```python
from build123d import *

# Parameters (mm, degrees)
SKETCH1_W                      = 260
SKETCH1_H                      = 132
BOSS_EXTRUDE1_DEPTH            = 150
SHELL1_T                       = -12
SKETCH2_W                      = 270
SKETCH2_H                      = 160
SKETCH2_W_2                    = 260
SKETCH2_H_2                    = 132
BOSS_EXTRUDE2_DEPTH            = 10
SKETCH3_R                      = 3.5
CUT_EXTRUDE1_DEPTH             = 10
CUT_EXTRUDE2_REACH             = 251.08
SKETCH4_R                      = 21
CHAMFER1_SIZE                  = 1
FILLET1_R                      = 2
M5_CLEARANCE_HOLE1_D           = 5.3
M5_CLEARANCE_HOLE1_CSINK_D     = 5.35
M5_CLEARANCE_HOLE1_CSINK_ANGLE = 90


with BuildPart() as part:
    # Sketch1 → Boss-Extrude1 (new body)
    with BuildSketch(Plane(origin=(0, 0, 0), x_dir=(1, 0, 0), z_dir=(0, 1, 0))):
        Rectangle(SKETCH1_W, SKETCH1_H)
    extrude(amount=BOSS_EXTRUDE1_DEPTH)

    # Shell1
    shell1_openings = [part.faces().sort_by_distance(p)[0] for p in [
        (0, 150, 0),
    ]]
    offset(amount=SHELL1_T, openings=shell1_openings, kind=Kind.INTERSECTION)

    # Sketch2 → Boss-Extrude2 (add)
    with BuildSketch(Plane(origin=(0, 150, 0), x_dir=(1, 0, 0), z_dir=(0, 1, 0))):
        Rectangle(SKETCH2_W, SKETCH2_H)
        Rectangle(SKETCH2_W_2, SKETCH2_H_2, mode=Mode.SUBTRACT)
    extrude(amount=-BOSS_EXTRUDE2_DEPTH)

    # Sketch3 → Cut-Extrude1 (cut)
    with BuildSketch(Plane(origin=(0, 150, 0), x_dir=(1, 0, 0), z_dir=(0, 1, 0))):
        with Locations(Location((-125, 73, 0), (0, 0, 270))):
            Circle(SKETCH3_R)
        with Locations(Location((128, 73, 0), (0, 0, 270))):
            Circle(SKETCH3_R)
        with Locations(Location((128, -73, 0), (0, 0, 270))):
            Circle(SKETCH3_R)
        with Locations(Location((-125, -73, 0), (0, 0, 270))):
            Circle(SKETCH3_R)
    extrude(amount=-CUT_EXTRUDE1_DEPTH, mode=Mode.SUBTRACT)

    # Cut-Extrude2: up to this face of the body (flat: up to its plane)
    cut_extrude2_end = Plane(part.part.faces().sort_by_distance((0, 70, -66))[0])
    # Sketch4 → Cut-Extrude2 (cut, up to the picked face)
    with BuildSketch(Plane.XY.offset(66), mode=Mode.PRIVATE) as cut_extrude2_sk1:
        with Locations((-75, 100)):
            Circle(SKETCH4_R)
    cut_extrude2_tool1 = split(extrude(cut_extrude2_sk1.sketch, amount=-CUT_EXTRUDE2_REACH, mode=Mode.PRIVATE), bisect_by=cut_extrude2_end, keep=Keep.BOTH, mode=Mode.PRIVATE)
    # Sketch4 → Cut-Extrude2 (cut, up to the picked face)
    with BuildSketch(Plane.XY.offset(66), mode=Mode.PRIVATE) as cut_extrude2_sk2:
        with Locations((25, 100)):
            Circle(SKETCH4_R)
    cut_extrude2_tool2 = split(extrude(cut_extrude2_sk2.sketch, amount=-CUT_EXTRUDE2_REACH, mode=Mode.PRIVATE), bisect_by=cut_extrude2_end, keep=Keep.BOTH, mode=Mode.PRIVATE)
    add(cut_extrude2_tool1.solids().sort_by(Axis((-75, 100, 66), (0, 0, -1)))[0], mode=Mode.SUBTRACT)
    add(cut_extrude2_tool2.solids().sort_by(Axis((25, 100, 66), (0, 0, -1)))[0], mode=Mode.SUBTRACT)

    # Chamfer1
    chamfer1_edges = [part.edges().sort_by_distance(p)[0] for p in [
        (-125, 150, 69.5),
        (128, 150, 69.5),
        (128, 150, -76.5),
        (-125, 150, -76.5),
    ]]
    chamfer(chamfer1_edges, length=CHAMFER1_SIZE)

    # Fillet1
    fillet1_edges = [part.edges().sort_by_distance(p)[0] for p in [
        (-118, 12, 0),
        (-118, 81, -54),
        (0, 12, 54),
        (-118, 81, 54),
        (118, 12, 0),
        (118, 81, 54),
        (0, 12, -54),
        (118, 81, -54),
    ]]
    fillet(fillet1_edges, radius=FILLET1_R)

    # M5 Clearance Hole1 (through all)
    with Locations(Plane.XY.offset(66)):
        with Locations((55, 100), (-75, 130), (-105, 100), (-75, 70), (-45, 100), (25, 130), (-5, 100), (25, 70)):
            CounterSinkHole(M5_CLEARANCE_HOLE1_D / 2, M5_CLEARANCE_HOLE1_CSINK_D / 2, counter_sink_angle=M5_CLEARANCE_HOLE1_CSINK_ANGLE)


solid = part.part
```
CAD build for the part. Positions are in the model's coordinates, mm. A direction names the side the tool comes from. Coordinates: 2 decimals unless noted, no trailing zeros. Write each loop counter-clockwise with the first axis right and the second up, starting at its lowest first coordinate (ties: lowest second). Pieces come first, ordered by that corner, then holes. Notation, with made-up numbers: (-40, 72) -> (7, 72) arc R9 cw to (7, 81) -> close; hole circle Ø10 at (-4, -20). An arc over 180 degrees is marked (long way). Return JSON: item names as keys, results as strings. Group by question number.
Q1. Cut at C-C, the plane z = -61. State how many separate pieces and enclosed holes the cut face has, then the cut area to 3 significant figures.
Q2. Flat gauge pins, fed straight in: pin 1 (1 mm diameter, centred on x = -72.5, y = 77, fed in from -Z); pin 2 (10 mm diameter, centred on y = 60, z = -47.5, fed in from -X); pin 3 (1 mm diameter, centred on x = -65, z = 10.5, fed in from +Y). Where does each tip first touch, or does it go through?
Q3. Cut at A-A, the plane z = 73. Give the cut face in (x, y), then the cut area to 3 significant figures.
Q4. Pull direction X, two halves, no side cores. Call faces 3 (the face through (-1.9, 150, -54.5)), 4 (the face through (130, 69, 1)), 5 (the face through (-135, 145, 1)), 6 (the face through (-104.43, 97.41, 59.9)): released by +X, released by -X, zero draft, split by the parting line, or undercut.
Q5. Cut at D-D, the plane x = 38.5. Give the cut face in (y, z), then the cut area to 3 significant figures.
Q6. Which spindle directions (+Z, -Z, +X, -X, +Y, -Y) get a long thin tool onto all of the face, cutting with end or side? Do faces 1 (the face through (118, 81, 1)), 2 (the face through (-76.223, 67.649, -60.084)). Say none if no direction does.
Q7. Cut at B-B, the plane y = 23.5. Give the cut face in (x, z).
Q8. Drill centre lines: line 1 (Y direction, x = -75, z = -60.25); line 2 (X direction, y = 73.5, z = -19); line 3 (Z direction, x = -98.5, y = 116.5). Where is each one in solid material? Low to high.
Returned:
{
 "1": {"separate pieces": "1", "enclosed holes": "10", "area": "36,200 mm2"},
 "2": {"pin 1": "stops at z = -66", "pin 2": "stops at x = -130", "pin 3": "stops at y = 12"},
 "3": {"outline": "(-135, 140) -> (-128.5, 140) -> (-128.5, 149) -> (-129.5, 150) -> (-135, 150) -> close; (-121.5, 140) -> (124.5, 140) -> (124.5, 149) -> (123.5, 150) -> (-120.5, 150) -> (-121.5, 149) -> close; (131.5, 140) -> (135, 140) -> (135, 150) -> (132.5, 150) -> (131.5, 149) -> close", "area": "2,560 mm2"},
 "4": {"face 3": "zero draft", "face 4": "released by +X", "face 5": "released by -X", "face 6": "undercut"},
 "5": {"outline": "(0, -66) -> (83.91, -66) -> (83.91, -54) -> (14, -54) arc R2 cw to (12, -52) -> (12, 52) arc R2 cw to (14, 54) -> (83.91, 54) -> (83.91, 66) -> (0, 66) -> close; (116.09, -66) -> (140, -66) -> (140, -80) -> (150, -80) -> (150, -54) -> (116.09, -54) -> close; (116.09, 54) -> (150, 54) -> (150, 80) -> (140, 80) -> (140, 66) -> (116.09, 66) -> close", "area": "4,410 mm2"},
 "6": {"face 1": "+Y", "face 2": "+Z, -Z"},
 "7": {"outline": "(-130, -66) -> (130, -66) -> (130, 66) -> (-130, 66) -> close; hole (-118, -52) arc R2 ccw to (-116, -54) -> (116, -54) arc R2 ccw to (118, -52) -> (118, 52) arc R2 ccw to (116, 54) -> (-116, 54) arc R2 ccw to (-118, 52) -> close"},
 "8": {"line 1": "y = 0 to 67.35, 72.65 to 79, 121 to 127.35, 132.65 to 150", "line 2": "x = -130 to -118, 118 to 130", "line 3": "z = -66 to -54, 54 to 66"}
}
